from build123d import *

# Parameters (mm, degrees)
BOX009_W          = 15
BOX009_H          = 1.6
BOX009_DEPTH      = 10.5
CYLINDER019_R     = 2.9
CYLINDER019_DEPTH = 10.5
CYLINDER018_R     = 4.5
CYLINDER018_DEPTH = 7
CYLINDER017_R     = 13.5
CYLINDER017_DEPTH = 10.8
CYLINDER016_R     = 15.1
CYLINDER016_DEPTH = 10.8
CHAMFER006_SIZE   = 1.6
CHAMFER007_SIZE   = 1.6
CHAMFER008_SIZE   = 1.6


with BuildPart() as obj1:
    # Box009 → Box009 (new body)
    with BuildSketch(Plane(origin=(123, 18.3, 1.6), x_dir=(1, 0, 0), z_dir=(0, 0, 1))):
        with Locations((7.5, 0.8)):
            Rectangle(BOX009_W, BOX009_H)
    extrude(amount=BOX009_DEPTH)


with BuildPart() as zylinder019:
    # Cylinder019 → Cylinder019 (new body)
    with BuildSketch(Plane(origin=(130, 19.1, 1.6), x_dir=(1, 0, 0), z_dir=(0, 0, 1))):
        Circle(CYLINDER019_R)
    extrude(amount=CYLINDER019_DEPTH)


with BuildPart() as cut009:
    # Cylinder018 → Cylinder018 (new body)
    with BuildSketch(Plane(origin=(130, 19.1, 0), x_dir=(1, 0, 0), z_dir=(0, 0, 1))):
        Circle(CYLINDER018_R)
    extrude(amount=CYLINDER018_DEPTH)

    # Cut009: cut Zylinder019
    add(zylinder019.part, mode=Mode.SUBTRACT)


with BuildPart() as zylinder017:
    # Cylinder017 → Cylinder017 (new body)
    with BuildSketch(Plane(origin=(130, 19.1, 1.6), x_dir=(1, 0, 0), z_dir=(0, 0, 1))):
        Circle(CYLINDER017_R)
    extrude(amount=CYLINDER017_DEPTH)


with BuildPart() as knob:
    # Cylinder016 → Cylinder016 (new body)
    with BuildSketch(Plane(origin=(130, 19.1, 0), x_dir=(1, 0, 0), z_dir=(0, 0, 1))):
        Circle(CYLINDER016_R)
    extrude(amount=CYLINDER016_DEPTH)

    # Cut008: cut Zylinder017
    add(zylinder017.part, mode=Mode.SUBTRACT)

    # Chamfer006
    chamfer006_edges = [knob.edges().sort_by_distance(p)[0] for p in [
        (116.5, 19.1, 1.6),
    ]]
    chamfer(chamfer006_edges, length=CHAMFER006_SIZE)

    # Chamfer007
    chamfer007_edges = [knob.edges().sort_by_distance(p)[0] for p in [
        (114.9, 19.1, 0),
    ]]
    chamfer(chamfer007_edges, length=CHAMFER007_SIZE)

    # Fusion011: union Cut009
    add(cut009.part)

    # Chamfer008
    chamfer008_edges = [knob.edges().sort_by_distance(p)[0] for p in [
        (125.5, 19.1, 1.6),
    ]]
    chamfer(chamfer008_edges, length=CHAMFER008_SIZE)

    # Cut010: cut obj1
    add(obj1.part, mode=Mode.SUBTRACT)


solid = knob.part
Verification items for the finished model (mm, model axes). A direction names the side the tool comes from. Give positions to 0.01 mm unless a question says otherwise; leave off trailing zeros. Loops run counter-clockwise (first coordinate to the right, second up) from the corner with the lowest first, then second, coordinate; pieces in that order, holes last.
1) Sectioned sample at B-B, the plane y = 19.1. Enter the section's corners in (x, z), then the cut area to 3 significant figures.
2) Thickness scan on line 1 along Y through (x, z) = (130, 6.25); line 2 along Y through (x, z) = (130, 7.5); line 3 along Y through (x, z) = (126, 2.75). Record the ranges inside material, lowest first.
3) Sectioned sample at D-D, the plane z = 9.5. Enter the section's corners in (x, y).
4) Sectioned sample at C-C, the plane x = 130. Enter the section's corners in (y, z).
5) Depth check by flat-ended pin: pin 1 Ø4 at (x, z) = (139.5, 7.5) entering from -Y; pin 2 Ø12 at (x, y) = (134, 15) entering from +Z; pin 3 Ø4 at (x, y) = (121.5, 26.5) entering from -Z; pin 4 Ø1 at (x, z) = (140, 1.5) entering from +Y. Enter the tip coordinate at first touch or a pass-through.
6) Set-up check for faces 1 (the flat face through (130, 19, 0)), 2 (the conical face through (130.1, 14.3, 2.9)): record each of +Z, -Z, +X, -X, +Y, -Y from which the full face is reachable in a straight line by a thin tool's end or side.
7) Draft check along Y on faces 3 (the flat face through (119, 11, 10.8)), 4 (the flat face through (134, 19.9, 4)), 5 (the cylindrical face through (118.871, 29.305, 6.136)). Enter one of: pulls with the +Y half, pulls with the -Y half, needs draft (parallel to the pull), parting line crosses it, or undercut.
8) Sectioned sample at A-A, the plane z = 6.5. Enter the section's corners in (x, y).
Answers:
1. outline: (114.9, 1.6) - (116.5, 0) - (143.5, 0) - (145.1, 1.6) - (145.1, 10.8) - (143.5, 10.8) - (143.5, 3.2) - (141.9, 1.6) - (118.1, 1.6) - (116.5, 3.2) - (116.5, 10.8) - (114.9, 10.8) - close
1. area: 77.8 mm2
2. line 1: y = 4 to 5.6, 14.6 to 16.2, 22 to 23.6, 32.6 to 34.2
2. line 2: y = 4 to 5.6, 32.6 to 34.2
2. line 3: y = 4.54 to 6.68, 16.18 to 18.3, 19.9 to 22.02, 31.52 to 33.66
3. outline: circle Ø30.2 at (130, 19.1); hole circle Ø27 at (130, 19.1)
4. outline: (4, 1.6) - (5.6, 0) - (32.6, 0) - (34.2, 1.6) - (34.2, 10.8) - (32.6, 10.8) - (32.6, 3.2) - (31, 1.6) - (25.2, 1.6) - (23.6, 3.2) - (23.6, 7) - (22, 7) - (22, 1.6) - (16.2, 1.6) - (16.2, 7) - (14.6, 7) - (14.6, 3.2) - (13, 1.6) - (7.2, 1.6) - (5.6, 3.2) - (5.6, 10.8) - (4, 10.8) - close
5. pin 1: stops at y = 5.99
5. pin 2: stops at z = 7
5. pin 3: stops at z = 0
5. pin 4: stops at y = 30.83
6. face 1: -Z, +X, -X, +Y, -Y
6. face 2: +Z
7. face 3: needs draft
7. face 4: undercut
7. face 5: parting line crosses it
8. outline: circle Ø30.2 at (130, 19.1); (125.57, 18.3) arc R4.5 ccw to (134.43, 18.3) - (132.79, 18.3) arc R2.9 cw to (127.21, 18.3) - close; (125.57, 19.9) - (127.21, 19.9) arc R2.9 cw to (132.79, 19.9) - (134.43, 19.9) arc R4.5 ccw to start; hole circle Ø27 at (130, 19.1)
